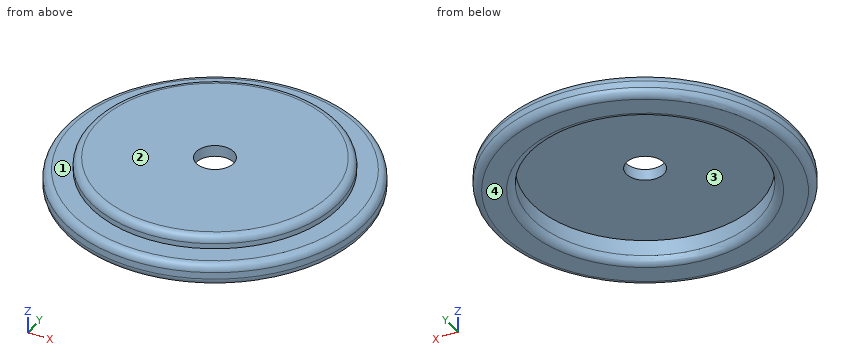
from build123d import *

# Parameters (mm, degrees)
F2_R     = 1
F3_R     = 2.5
F4_DEPTH = 1.501


# Not quite as in the source:
# - a feature names something its author has since deleted; it is built from what else it names


with BuildPart() as f1:
    # F0 (on Front) → F1 (revolve)
    with BuildSketch(Plane.XZ):
        Polygon((15.1, 3.1), (15.1, 0), (20, 0), (20, 2.9), (16.5, 2.9), (16.5, 4.6), (0, 4.6), (0, 3.1), align=None)
    revolve(axis=Axis((0, 0, 3.0650238041), (0, 0, -1)))

    # F2
    f2_edges = [f1.edges().sort_by_distance(p)[0] for p in [
        (-15.1, 0, 0),
        (-20, 0, 0),
        (-16.5, 0, 4.6),
        (-20, 0, 2.9),
    ]]
    fillet(f2_edges, radius=F2_R)

    # F3 (on face) → F4 (cut, through all)
    with BuildSketch(Plane(origin=(0, 0, 3.1), x_dir=(1, 0, 0), z_dir=(0, 0, -1))):
        Circle(F3_R)
    extrude(amount=-F4_DEPTH, mode=Mode.SUBTRACT)


solid = f1.part
Can you work these out from the model? Positions are in its coordinate system, mm. Face numbers are marked on the shaded views. A direction names the side the tool comes from. Coordinates: 2 decimals unless noted, no trailing zeros. Write each loop counter-clockwise with the first axis right and the second up, starting at its lowest first coordinate (ties: lowest second). Pieces come first, ordered by that corner, then holes. Notation, with made-up numbers: (-10, 58.5) - (23, 58.5) arc R13 ccw to (23, 64.5) - close; hole circle Ø6 at (69, 53). An arc over 180 degrees is marked (long way). Return JSON: item names as keys, results as strings. Group by question number.
Item 1: Please list where these lines run through material, in increasing order: probe 1 along X at (y, z) = (0, 1.6); probe 2 along Y at (x, z) = (0, 3.7).
Item 2: I'm going to push flat-ended pins straight in: pin 1 Ø24 at (x, y) = (5, 4) entering from -Z; pin 2 Ø5 at (x, y) = (0.5, 9) entering from -Z; pin 3 Ø2 at (x, z) = (5, 3) entering from +Y; pin 4 Ø1.5 at (x, z) = (4, 3) entering from +Y. Where does each tip first touch, or does it pass through?
Item 3: We'd pull the mould along X, two halves only. Please class the marked faces 3 and 4: pulls with the +X half, pulls with the -X half, needs draft (parallel to the pull), parting line crosses it, or undercut.
Item 4: If we section it at A-A (x = 0): Write out the boundary of the cut face in (y, z).
Item 5: Which directions (+Z, -Z, +X, -X, +Y, -Y) give clear straight access to the entire face, cutting with the end or side of a thin tool? Please do the marked faces 1 and 2.
Return value:
{
 "1": {"probe 1": "x = -20 to -15.1, 15.1 to 20", "probe 2": "y = -16.49 to -2.5, 2.5 to 16.49"},
 "2": {"pin 1": "stops at z = 0", "pin 2": "stops at z = 3.1", "pin 3": "stops at y = 19.46", "pin 4": "stops at y = 19.56"},
 "3": {"face 3": "undercut", "face 4": "needs draft"},
 "4": {"outline": "(-20, 1) arc R1 ccw to (-19, 0) - (-16.1, 0) arc R1 ccw to (-15.1, 1) - (-15.1, 3.1) - (-2.5, 3.1) - (-2.5, 4.6) - (-15.5, 4.6) arc R1 ccw to (-16.5, 3.6) - (-16.5, 2.9) - (-19, 2.9) arc R1 ccw to (-20, 1.9) - close; (2.5, 3.1) - (15.1, 3.1) - (15.1, 1) arc R1 ccw to (16.1, 0) - (19, 0) arc R1 ccw to (20, 1) - (20, 1.9) arc R1 ccw to (19, 2.9) - (16.5, 2.9) - (16.5, 3.6) arc R1 ccw to (15.5, 4.6) - (2.5, 4.6) - close"},
 "5": {"face 1": "+Z", "face 2": "+Z, +X, -X, +Y, -Y"}
}
